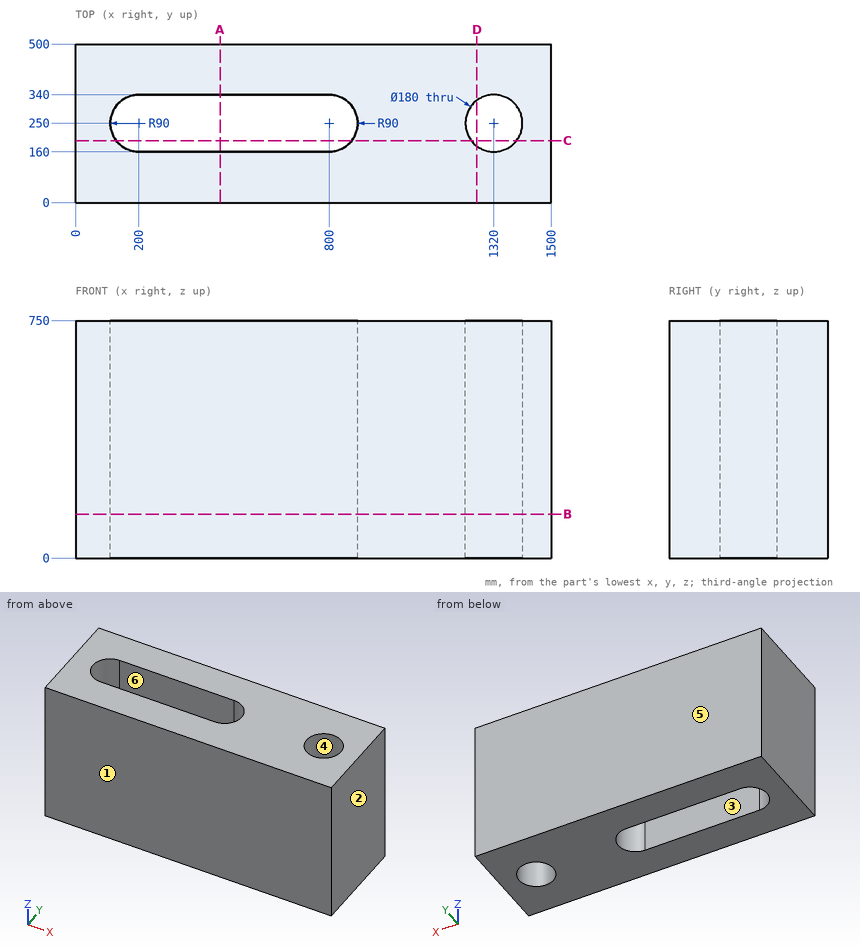
Job drawing, mm, ordinate dimensions from the low corner. One solid piece. A direction names the side the tool comes from. Give positions to 0.01 mm unless a question says otherwise; leave off trailing zeros. Loops run counter-clockwise (first coordinate to the right, second up) from the corner with the lowest first, then second, coordinate; pieces in that order, holes last.
Item 1: Drill centre lines: line 1 (Y direction, x = 756.5, z = 522.5); line 2 (X direction, y = 235, z = 683.5); line 3 (X direction, y = 211.5, z = 646.5). Where is each one in solid material? Low to high.
Answers follow:
line 1: y = 0 to 160, 340 to 500
line 2: x = 0 to 111.26, 888.74 to 1231.26, 1408.74 to 1500
line 3: x = 0 to 118.65, 881.35 to 1238.65, 1401.35 to 1500
Item 2: Slice it at A-A, the plane x = 456. List the corners of the cut face in (y, z).
Answers follow:
outline: (0, 0) - (160, 0) - (160, 750) - (0, 750) - close; (340, 0) - (500, 0) - (500, 750) - (340, 750) - close
Item 3: Slice it at C-C, the plane y = 195.5. List the corners of the cut face in (x, z).
Answers follow:
outline: (0, 0) - (128.38, 0) - (128.38, 750) - (0, 750) - close; (871.62, 0) - (1248.38, 0) - (1248.38, 750) - (871.62, 750) - close; (1391.62, 0) - (1500, 0) - (1500, 750) - (1391.62, 750) - close
Item 4: Pull direction X, two halves, no side cores. Call the marked faces 1, 2, 3 and 4: released by +X, released by -X, zero draft, split by the parting line, or undercut.
Answers follow:
face 1: zero draft
face 2: released by +X
face 3: undercut
face 4: undercut
Item 5: Which spindle directions (+Z, -Z, +X, -X, +Y, -Y) get a long thin tool onto all of the face, cutting with end or side? Do the marked faces 5 and 6. Say none if no direction does.
Answers follow:
face 5: +Z, -Z, +X, -X, +Y
face 6: +Z, -Z
Item 6: Slice it at B-B, the plane z = 139. List the corners of the cut face in (x, y), and give its area (3 significant figures).
Answers follow:
outline: (0, 0) - (1500, 0) - (1500, 500) - (0, 500) - close; hole (200, 160) - (800, 160) arc R90 ccw to (800, 340) - (200, 340) arc R90 ccw to start; hole circle Ø180 at (1320, 250)
area: 591,000 mm2
Item 7: Slice it at D-D, the plane x = 1266. List the corners of the cut face in (y, z).
Answers follow:
outline: (0, 0) - (178, 0) - (178, 750) - (0, 750) - close; (322, 0) - (500, 0) - (500, 750) - (322, 750) - close
